from build123d import *

# Parameters (mm, degrees)
F1_DEPTH = 9.525
F2_R     = 5.08
F3_T     = -2.54
F4_R     = 15.875
F5_DEPTH = 25.4


with BuildPart() as f1:
    # F0 (on Front) → F1 (new body)
    with BuildSketch(Plane.XZ):
        with BuildLine():
            Line((31.75, 101.6), (-31.75, 101.6))
            ThreePointArc((-31.75, 101.6), (-40.730256, 97.880256), (-44.45, 88.9))
            Line((-44.45, 88.9), (-44.45, -88.9))
            ThreePointArc((-44.45, -88.9), (-40.730256, -97.880256), (-31.75, -101.6))
            Line((-31.75, -101.6), (31.75, -101.6))
            ThreePointArc((31.75, -101.6), (40.730256, -97.880256), (44.45, -88.9))
            Line((44.45, -88.9), (44.45, 88.9))
            ThreePointArc((44.45, 88.9), (40.730256, 97.880256), (31.75, 101.6))
        make_face()
    extrude(amount=F1_DEPTH)

    # F2
    f2_edges = [f1.edges().sort_by_distance(p)[0] for p in [
        (0, 0, 101.6),
        (-40.730256, 0, 97.880256),
        (-44.45, 0, 0),
        (-40.730256, 0, -97.880256),
        (0, 0, -101.6),
        (40.730256, 0, -97.880256),
        (44.45, 0, 0),
        (40.730256, 0, 97.880256),
    ]]
    fillet(f2_edges, radius=F2_R)

    # F3
    f3_openings = [f1.faces().sort_by_distance(p)[0] for p in [
        (0, -9.525, 0),
    ]]
    offset(amount=F3_T, openings=f3_openings)

    # F4 (on face) → F5 (cut)
    with BuildSketch(Plane.XZ.offset(2.54)):
        with Locations((0, 43.90662)):
            Circle(F4_R)
    extrude(amount=-F5_DEPTH, mode=Mode.SUBTRACT)


solid = f1.part
Can you work these out from the model? Positions are in its coordinate system, mm. A direction names the side the tool comes from. Coordinates: 2 decimals unless noted, no trailing zeros. Loops run counter-clockwise (first coordinate to the right, second up) from the corner with the lowest first, then second, coordinate; pieces in that order, holes last. Notation, with made-up numbers: (2, 67.25) - (25, 67.25) arc R23 ccw to (25, 82.25) - close; hole circle Ø6 at (89, 27.5). An arc over 180 degrees is marked (long way). Answer as a JSON object with one key per item and string values. Group by question number.
Item 1: If we section it at A-A (x = 0): List the corners of the cut face in (y, z) for me (3 decimals), plus the area to 3 significant figures.
Item 2: If we section it at C-C (x = 19): List the corners of the cut face in (y, z) for me (3 decimals).
Item 3: On a 3-axis mill with a long thin cutter (end or side, diameter ignored), from which of +Z, -Z, +X, -X, +Y, -Y can I reach the whole of each face in a straight line? I mean faces 1 (the face through (-1, 0, 1)), 2 (the face through (38.855, -7.271, -96.163)). Say none if no direction works.
Item 4: If I drill on L1, parallel to X at y = -6, z = 20.5; L2, parallel to Y at x = 6.5, z = -4.5; L3, parallel to Z at x = 5.5, y = -7.25, over which ranges is the centre line in solid material (lowest first)? Write a range as from..to.
Item 5: If we section it at B-B (z = 77.5): List the corners of the cut face in (x, y) for me (3 decimals), plus the area to 3 significant figures.
Item 6: If we mould it in two halves opening along Z, with no side actions, what happens to faces 3 (the face through (40.83, -7.27, 97.78)), 4 (the face through (41.91, -7, -1)), 5 (the face through (-43.001, -1.528, -1.245))? For each: released by +Z, released by -Z, zero draft, split by the parting line, or undercut.
Returned:
{
 "1": {"outline": "(-9.525, -101.6) - (-5.08, -101.6) arc R5.08 ccw to (0, -96.52) - (0, 28.032) - (-2.54, 28.032) - (-2.54, -96.52) arc R2.54 cw to (-5.08, -99.06) - (-9.525, -99.06) - close; (-9.525, 99.06) - (-5.08, 99.06) arc R2.54 cw to (-2.54, 96.52) - (-2.54, 59.782) - (0, 59.782) - (0, 96.52) arc R5.08 ccw to (-5.08, 101.6) - (-9.525, 101.6) - close", "area": "463 mm²"},
 "2": {"outline": "(-9.525, -101.6) - (-5.08, -101.6) arc R5.08 ccw to (0, -96.52) - (0, 96.52) arc R5.08 ccw to (-5.08, 101.6) - (-9.525, 101.6) - (-9.525, 99.06) - (-5.08, 99.06) arc R2.54 cw to (-2.54, 96.52) - (-2.54, -96.52) arc R2.54 cw to (-5.08, -99.06) - (-9.525, -99.06) - close"},
 "3": {"face 1": "+Z, -Z, +X, -X, +Y", "face 2": "-Y"},
 "4": {"L1": "x = -44.45..-41.91, 41.91..44.45", "L2": "y = -2.54..0", "L3": "z = -101.6..-99.06, 99.06..101.6"},
 "5": {"outline": "(-44.45, -9.525) - (-41.91, -9.525) - (-41.91, -5.08) arc R2.54 cw to (-39.37, -2.54) - (39.37, -2.54) arc R2.54 cw to (41.91, -5.08) - (41.91, -9.525) - (44.45, -9.525) - (44.45, -5.08) arc R5.08 ccw to (39.37, 0) - (-39.37, 0) arc R5.08 ccw to (-44.45, -5.08) - close", "area": "253 mm²"},
 "6": {"face 3": "released by +Z", "face 4": "undercut", "face 5": "zero draft"}
}
